Part model, mm, in its own coordinate system. Face numbers are marked on the shaded views. A direction names the side the tool comes from. Round coordinates to 2 decimals unless told otherwise and drop trailing zeros. Order: outer loops, then holes, each group sorted by start corner. A loop starts at its lowest first (then second) coordinate and runs counter-clockwise, first axis right, second up. Notation, with made-up numbers: (-6, -28) - (0, -28) arc R21 ccw to (0, 3) - close; hole circle Ø6 at (-37.5, 49.5). An arc over 180 degrees is marked (long way). Return JSON: item names as keys, results as strings. Group by question number.
Item 1: Probe probe 1 along Z at (x, y) = (-4, 1); probe 2 along Z at (x, y) = (-9, 6.5); probe 3 along X at (y, z) = (6, 6.75). List the from-to ranges inside material, lowest first.
Item 2: Tool access for the marked faces 1, 2, 3, 4 and 5: list every direction of +Z, -Z, +X, -X, +Y, -Y with a clear straight run to the whole face (end or side of a thin tool).
Item 3: Saw through at B-B on z = 24.25. List the corners of the cut face in (x, y), and give its area (3 significant figures).
Item 4: Drop flat-ended pins along their axis: pin 1 (4.5 mm diameter, centred on y = 5, z = 21, fed in from -X); pin 2 (2.5 mm diameter, centred on x = 9, y = 1.5, fed in from -Z); pin 3 (2.5 mm diameter, centred on x = 9.3, y = 3.97, fed in from +Z); pin 4 (2 mm diameter, centred on x = -17, z = 7.5, fed in from +Y). Give the stop position or say it passes through.
Item 5: Saw through at A-A on z = 3.75. List the corners of the cut face in (x, y), and give its area (3 significant figures).
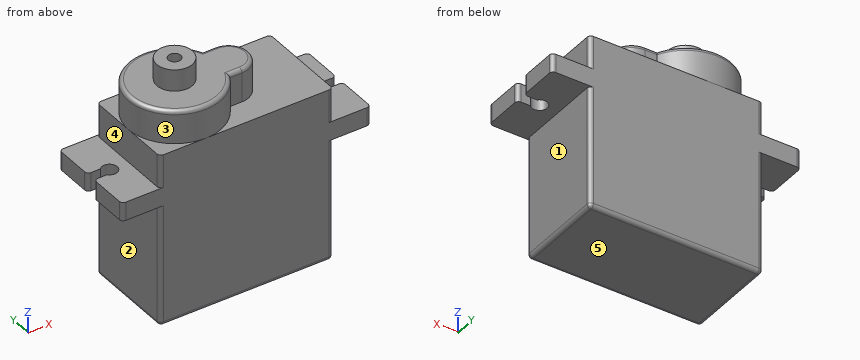
```python
from build123d import *

# Parameters (mm, degrees)
SKETCH2_W                = 22.5
SKETCH2_H                = 12
BOSS_EXTRUDE1_DEPTH      = 22.5
SKETCH3_W                = 2.4
SKETCH3_H                = 12
BOSS_EXTRUDE2_DEPTH      = 4.9
BOSS_EXTRUDE2_DEPTH_BACK = 27.4
CUT_EXTRUDE1_REACH       = 20.2
SKETCH4_R                = 1
SKETCH5_R                = 6
BOSS_EXTRUDE3_DEPTH      = 4.3
SKETCH6_R                = 2.3
BOSS_EXTRUDE4_DEPTH      = 2.8
SKETCH7_R                = 0.8
CUT_EXTRUDE2_DEPTH       = 7
CUT_EXTRUDE3_REACH       = 20.2
SKETCH8_W                = 4.668208072
SKETCH8_H                = 1.3
SKETCH8_W_2              = 4.280898206
BOSS_EXTRUDE6_DEPTH      = 4.3
FILLET1_R                = 0.5


with BuildPart() as part:
    # Sketch2 → Boss-Extrude1 (new body)
    with BuildSketch(Plane.XY):
        with Locations((-4.403809909, 3.974212835)):
            Rectangle(SKETCH2_W, SKETCH2_H)
    extrude(amount=BOSS_EXTRUDE1_DEPTH)

    # Sketch3 → Boss-Extrude2 (add, two sides)
    with BuildSketch(Plane(origin=(6.846190091, 0, 0), x_dir=(0, 0, -1), z_dir=(1, 0, 0))) as boss_extrude2_sk:
        with Locations((-17, 3.974212835)):
            Rectangle(SKETCH3_W, SKETCH3_H)
    extrude(amount=BOSS_EXTRUDE2_DEPTH)
    extrude(boss_extrude2_sk.sketch, amount=-BOSS_EXTRUDE2_DEPTH_BACK)

    # Sketch4 → Cut-Extrude1 (cut, up to next)
    with BuildSketch(Plane.XY.offset(18.2), mode=Mode.PRIVATE) as cut_extrude1_sk1:
        with Locations((9.296190091, 3.974212835)):
            Circle(SKETCH4_R)
    cut_extrude1_tool1 = extrude(cut_extrude1_sk1.sketch, amount=-CUT_EXTRUDE1_REACH, mode=Mode.PRIVATE) & part.part
    add(cut_extrude1_tool1.solids().sort_by_distance((9.29619, 3.974213, 18.2))[0], mode=Mode.SUBTRACT)
    # Sketch4 → Cut-Extrude1 (cut, up to next)
    with BuildSketch(Plane.XY.offset(18.2), mode=Mode.PRIVATE) as cut_extrude1_sk2:
        with Locations((-18.103809909, 3.974212835)):
            Circle(SKETCH4_R)
    cut_extrude1_tool2 = extrude(cut_extrude1_sk2.sketch, amount=-CUT_EXTRUDE1_REACH, mode=Mode.PRIVATE) & part.part
    add(cut_extrude1_tool2.solids().sort_by_distance((-18.10381, 3.974213, 18.2))[0], mode=Mode.SUBTRACT)

    # Sketch5 → Boss-Extrude3 (add)
    with BuildSketch(Plane.XY.offset(22.5)):
        with Locations((-9.653809909, 3.974212835)):
            Circle(SKETCH5_R)
    extrude(amount=BOSS_EXTRUDE3_DEPTH)

    # Sketch6 → Boss-Extrude4 (add)
    with BuildSketch(Plane.XY.offset(26.8)):
        with Locations((-9.653809909, 3.974212835)):
            Circle(SKETCH6_R)
    extrude(amount=BOSS_EXTRUDE4_DEPTH)

    # Sketch7 → Cut-Extrude2 (cut)
    with BuildSketch(Plane.XY.offset(29.6)):
        with Locations((-9.653809909, 3.974212835)):
            Circle(SKETCH7_R)
    extrude(amount=-CUT_EXTRUDE2_DEPTH, mode=Mode.SUBTRACT)

    # Sketch8 → Cut-Extrude3 (cut, up to next)
    with BuildSketch(Plane.XY.offset(18.2), mode=Mode.PRIVATE) as cut_extrude3_sk1:
        with Locations((-20.553809909, 3.974212835)):
            Rectangle(SKETCH8_W, SKETCH8_H)
    cut_extrude3_tool1 = extrude(cut_extrude3_sk1.sketch, amount=-CUT_EXTRUDE3_REACH, mode=Mode.PRIVATE) & part.part
    add(cut_extrude3_tool1.solids().sort_by_distance((-20.55381, 3.974213, 18.2))[0], mode=Mode.SUBTRACT)
    # Sketch8 → Cut-Extrude3 (cut, up to next)
    with BuildSketch(Plane.XY.offset(18.2), mode=Mode.PRIVATE) as cut_extrude3_sk2:
        with Locations((11.746190091, 3.974212835)):
            Rectangle(SKETCH8_W_2, SKETCH8_H)
    cut_extrude3_tool2 = extrude(cut_extrude3_sk2.sketch, amount=-CUT_EXTRUDE3_REACH, mode=Mode.PRIVATE) & part.part
    add(cut_extrude3_tool2.solids().sort_by_distance((11.74619, 3.974213, 18.2))[0], mode=Mode.SUBTRACT)

    # Sketch9 → Boss-Extrude6 (add)
    with BuildSketch(Plane.XY.offset(22.5)):
        with BuildLine():
            Line((-2.653809909, 6.560409726), (-4.239792395, 6.560409726))
            Line((-4.239792395, 6.560409726), (-4.239792395, 1.388015944))
            Line((-4.239792395, 1.388015944), (-2.653809909, 1.388015944))
            ThreePointArc((-2.653809909, 1.388015944), (-0.067613018, 3.974212835), (-2.653809909, 6.560409726))
        make_face()
    extrude(amount=BOSS_EXTRUDE6_DEPTH)

    # Fillet1
    fillet1_edges = [part.edges().sort_by_distance(p)[0] for p in [
        (-15.653809909, 9.974212835, 7.9),
        (6.846190091, 9.974212835, 7.9),
        (6.846190091, -2.025787165, 7.9),
        (-15.653809909, -2.025787165, 7.9),
        (-20.553809909, 9.974212835, 17),
        (-20.553809909, -2.025787165, 17),
        (11.746190091, -2.025787165, 17),
        (11.746190091, 9.974212835, 17),
        (-4.403809909, 9.974212835, 0),
        (6.846190091, 3.974212835, 0),
        (-15.653809909, 3.974212835, 26.8),
        (-4.403809909, -2.025787165, 0),
        (-15.653809909, 3.974212835, 0),
        (-20.553809909, 3.324212835, 17),
        (-20.553809909, 4.624212835, 17),
        (-15.653809909, 9.974212835, 20.35),
        (6.846190091, 9.974212835, 20.35),
        (6.846190091, -2.025787165, 20.35),
        (-15.653809909, -2.025787165, 20.35),
        (11.746190091, 3.324212835, 17),
        (11.746190091, 4.624212835, 17),
        (-3.446801152, 1.388015944, 26.8),
        (-0.067613018, 3.974212835, 26.8),
        (-3.446801152, 6.560409726, 26.8),
    ]]
    fillet(fillet1_edges, radius=FILLET1_R)


solid = part.part
```
Filled in:
{
 "1": {"probe 1": "z = 0 to 22.5", "probe 2": "z = 0 to 26.8", "probe 3": "x = -15.65 to 6.85"},
 "2": {"face 1": "-Z, +X, +Y, -Y", "face 2": "-Z, -X, +Y, -Y", "face 3": "+Z", "face 4": "+Z, -X, +Y, -Y", "face 5": "-Z, +X, -X, +Y, -Y"},
 "3": {"outline": "(-4.24, 1.39) - (-2.65, 1.39) arc R2.59 ccw to (-2.65, 6.56) - (-4.24, 6.56) arc R6 ccw (long way) to start; hole circle Ø1.6 at (-9.65, 3.97)", "area": "128 mm^2"},
 "4": {"pin 1": "stops at x = -15.65", "pin 2": "stops at z = 15.8", "pin 3": "stops at z = 18.2", "pin 4": "passes through"},
 "5": {"outline": "(-15.65, -1.53) arc R0.5 ccw to (-15.15, -2.03) - (6.35, -2.03) arc R0.5 ccw to (6.85, -1.53) - (6.85, 9.47) arc R0.5 ccw to (6.35, 9.97) - (-15.15, 9.97) arc R0.5 ccw to (-15.65, 9.47) - close", "area": "270 mm^2"}
}
